Can you work these out from the model? Positions are in its coordinate system, mm. A direction names the side the tool comes from. Round coordinates to 2 decimals unless told otherwise and drop trailing zeros. Write each loop counter-clockwise with the first axis right and the second up, starting at its lowest first coordinate (ties: lowest second). Pieces come first, ordered by that corner, then holes. Notation, with made-up numbers: (-18.75, -24.5) - (39.25, -24.5) arc R14 cw to (39.25, -0.5) - close; hole circle Ø10 at (-6.75, 60.5). An arc over 180 degrees is marked (long way). One line per item, written item: value. Start each with the question number.
(1) I'm going to push a flat-ended pin straight in: pin 1 Ø5 at (y, z) = (-30, -16.5) entering from -X. Where does the tip first touch, or does it pass through?
(2) On a 3-axis mill with a long thin cutter (end or side, diameter ignored), from which of +Z, -Z, +X, -X, +Y, -Y can I reach the whole of each face in a straight line? I mean faces 4 (the face through (58, 1, 1)), 5 (the face through (24, -40, 1)), 6 (the face through (29, -1, 48)). Say none if no direction works.
(3) I want a section at D-D on x = 61.5. List the corners of the cut face in (y, z) for me.
(4) I want a section at A-A on x = 24.5. List the corners of the cut face in (y, z) for me.
(5) I want a section at C-C on z = 27.5. List the corners of the cut face in (x, y) for me.
(6) Thinking about a two-plate mould opening in Y: for faces 1 (the face through (64.16, 37.43, -32.42)), 2 (the face through (29, -48, 1)), 3 (the face through (29, -1, -48)), which applies, +Y half, -Y half, draft (parallel to the pull), parting line (faces both ways), or undercut?
(7) If I drill on L1, parallel to Z at x = 25, y = 36.5; L2, parallel to Z at x = 7, y = 14, over which ranges is the centre line in solid material (lowest first)? Write a range as from..to.
from build123d import *

# Parameters (mm, degrees)
ESQUISSE5_W        = 96
ESQUISSE5_H        = 96
ESQUISSE5_W_2      = 80
ESQUISSE5_H_2      = 80
BOSS_EXTRU_1_DEPTH = 48
ESQUISSE6_W        = 96
ESQUISSE6_H        = 96
BOSS_EXTRU_3_DEPTH = 10
ESQUISSE7_R        = 16.391900089
BOSS_EXTRU_4_DEPTH = 12.5
ESQUISSE8_R        = 18.5
ESQUISSE8_R_2      = 11.5
BOSS_EXTRU_5_DEPTH = 48
CHANFREIN2_SIZE2   = 48
CHANFREIN2_SIZE    = 4.199455849


with BuildPart() as part:
    # Esquisse5 → Boss.-Extru.1 (new body)
    with BuildSketch(Plane(origin=(0, 0, 0), x_dir=(0, 0, -1), z_dir=(1, 0, 0))):
        Rectangle(ESQUISSE5_W, ESQUISSE5_H)
        Rectangle(ESQUISSE5_W_2, ESQUISSE5_H_2, mode=Mode.SUBTRACT)
    extrude(amount=BOSS_EXTRU_1_DEPTH)

    # Esquisse6 → Boss.-Extru.3 (add)
    with BuildSketch(Plane(origin=(48, 0, 0), x_dir=(0, 0, -1), z_dir=(1, 0, 0))):
        Rectangle(ESQUISSE6_W, ESQUISSE6_H)
    extrude(amount=BOSS_EXTRU_3_DEPTH)

    # Esquisse7 → Boss.-Extru.4 (add)
    with BuildSketch(Plane(origin=(58, 0, 0), x_dir=(0, 0, -1), z_dir=(1, 0, 0))):
        with Locations((23.608099911, 23.608099911)):
            Circle(ESQUISSE7_R)
        with Locations((23.608099911, -23.608099911)):
            Circle(ESQUISSE7_R)
        with Locations((-23.608099911, -23.608099911)):
            Circle(ESQUISSE7_R)
        with Locations((-23.608099911, 23.608099911)):
            Circle(ESQUISSE7_R)
    extrude(amount=BOSS_EXTRU_4_DEPTH)

    # Esquisse8 → Boss.-Extru.5 (add)
    with BuildSketch(Plane.ZY):
        Circle(ESQUISSE8_R)
        Circle(ESQUISSE8_R_2, mode=Mode.SUBTRACT)
    extrude(amount=-BOSS_EXTRU_5_DEPTH)

    # Chanfrein2
    chanfrein2_edges = [part.edges().sort_by_distance(p)[0] for p in [
        (48, 0, -18.5),
    ]]
    chanfrein2_side = [part.faces().sort_by_distance(p)[0] for p in [
        (48, 0, -18.583989117),
    ]]
    chamfer(chanfrein2_edges, length=CHANFREIN2_SIZE - 0.0001, length2=CHANFREIN2_SIZE2 - 0.0001, reference=chanfrein2_side[0])  # a hair under: the kernel refuses the full size


solid = part.part
Established:
1. pin 1: x = 48
2. face 4: +X
2. face 5: -X
2. face 6: +Z, +X, -X, +Y, -Y
3. outline: circle Ø32.78 at (-23.61, -23.61); circle Ø32.78 at (-23.61, 23.61); circle Ø32.78 at (23.61, -23.61); circle Ø32.78 at (23.61, 23.61)
4. outline: (-48, -48) - (48, -48) - (48, 48) - (-48, 48) - close; circle Ø41.29 at (0, 0); hole (-40, -40) - (40, -40) - (40, 40) - (-40, 40) - close; hole circle Ø23 at (0, 0)
5. outline: (0, -48) - (58, -48) - (58, -39.53) - (70.5, -39.53) - (70.5, -7.68) - (58, -7.68) - (58, 7.68) - (70.5, 7.68) - (70.5, 39.53) - (58, 39.53) - (58, 48) - (0, 48) - (0, 40) - (48, 40) - (48, -40) - (0, -40) - close
6. face 1: undercut
6. face 2: -Y half
6. face 3: draft
7. L1: -48..-40, 40..48
7. L2: -48..-40, -13.01..13.01, 40..48
